Part model, mm, in its own coordinate system. A direction names the side the tool comes from. Coordinates: 2 decimals unless noted, no trailing zeros. Loops run counter-clockwise (first coordinate to the right, second up) from the corner with the lowest first, then second, coordinate; pieces in that order, holes last. Notation, with made-up numbers: M 41.5,50 L 57.5,50 A12 cw 57.5,64 Z; hole C 50,-14 d2. An arc over 180 degrees is marked long. Answer as a JSON object with one key per item and string values. Group by question number.
1. Drop flat-ended pins along their axis: pin 1 Ø8 at (x, y) = (2, -54) entering from +Z; pin 2 Ø3 at (x, y) = (-5, -12) entering from -Z; pin 3 Ø3.5 at (x, y) = (0.5, -91.5) entering from +Z; pin 4 Ø2 at (x, y) = (-6.5, -26.5) entering from +Z. Give the stop position or say it passes through.
2. Saw through at B-B on y = -98. Write the cut outline in (x, z), then the cut area to 3 significant figures.
3. Mould opens along Y. For faces 3 (the face through (0, -105, 0)), 4 (the face through (-1.5, -90, 7)), 5 (the face through (0, 0, 0)) say: released by +Y, released by -Y, zero draft, split by the parting line, or undercut.
4. 3-axis set-ups, long thin cutter, end or side, ignore diameter. For faces 1 (the face through (-1.951, -51.272, -8.786)), 2 (the face through (0, -90, 6)): which of +Z, -Z, +X, -X, +Y, -Y reach the whole face in a straight line?
5. Saw through at C-C on y = -66. Write the cut outline in (x, z), then the cut area to 3 significant figures.
6. Drill centre lines: L1, parallel to Z at x = -3, y = -84; L2, parallel to X at y = -85, z = -4.75. Where is each one in solid material? Low to high.
7. Saw through at A-A on x = 0. Write the cut outline in (y, z).
from build123d import *

# Parameters (mm, degrees)
F0_R     = 9
F1_DEPTH = 105
F2_SIZE  = 1
F5_DEPTH = 25


with BuildPart() as f1:
    # F0 (on Front) → F1 (new body)
    with BuildSketch(Plane.XZ):
        Circle(F0_R)
    extrude(amount=F1_DEPTH)

    # F2
    f2_edges = [f1.edges().sort_by_distance(p)[0] for p in [
        (-9, -105, 0),
    ]]
    chamfer(f2_edges, length=F2_SIZE)

    # F4 (on offset) → F5 (cut)
    with BuildSketch(Plane.XY.offset(6)):
        with BuildLine():
            ThreePointArc((1.5, -81), (0, -79.5), (-1.5, -81))
            Line((-1.5, -81), (-1.5, -99))
            ThreePointArc((-1.5, -99), (0, -100.5), (1.5, -99))
            Line((1.5, -99), (1.5, -81))
        make_face()
    extrude(amount=F5_DEPTH, mode=Mode.SUBTRACT)


solid = f1.part
Outcome:
{
 "1": {"pin 1": "stops at z = 9", "pin 2": "stops at z = -8.29", "pin 3": "stops at z = 8.87", "pin 4": "stops at z = 7.12"},
 "2": {"outline": "M -1.5,6 L -1.5,8.87 A9 ccw long 1.5,8.87 L 1.5,6 Z", "area": "246 mm²"},
 "3": {"face 3": "released by -Y", "face 4": "undercut", "face 5": "released by +Y"},
 "4": {"face 1": "+Y, -Y", "face 2": "+Z"},
 "5": {"outline": "C 0,0 d18", "area": "254 mm²"},
 "6": {"L1": "z = -8.49 to 8.49", "L2": "x = -7.64 to 7.64"},
 "7": {"outline": "M -105,-8 L -104,-9 L 0,-9 L 0,9 L -79.5,9 L -79.5,6 L -100.5,6 L -100.5,9 L -104,9 L -105,8 Z"}
}
